Geometry: final body of the model. Coordinates: model frame, mm. Face numbers are marked on the shaded views. A direction names the side the tool comes from. Give positions to 0.01 mm unless a question says otherwise; leave off trailing zeros. Order: outer loops, then holes, each group sorted by start corner. A loop starts at its lowest first (then second) coordinate and runs counter-clockwise, first axis right, second up. Notation, with made-up numbers: (75, 79) -> (126, 79) arc R14 ccw to (126, 101) -> close; hole circle Ø1 at (-30.75, 48.25). An arc over 180 degrees is marked (long way). Write item = value, one per line.
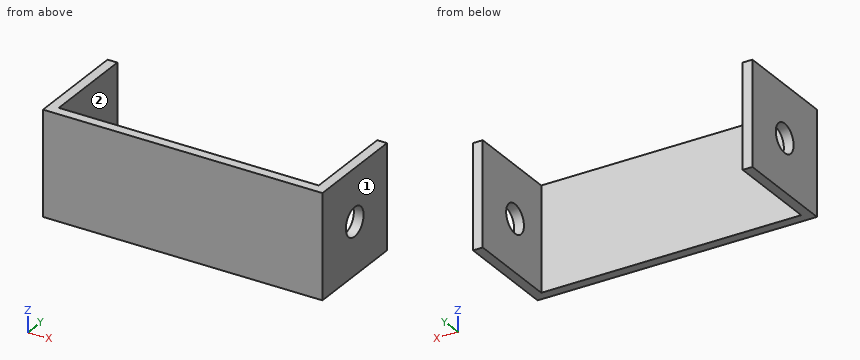
```python
from build123d import *

# Parameters (mm, degrees)
SKETCH1_W           = 127
SKETCH1_H           = 50.8
BOSS_EXTRUDE2_DEPTH = 4.7625
SKETCH3_W           = 4.7625
SKETCH3_H           = 50.8
BOSS_EXTRUDE3_DEPTH = 50.8
SKETCH4_R           = 6.985
CUT_EXTRUDE1_DEPTH  = 137.525


with BuildPart() as part:
    # Sketch1 → Boss-Extrude2 (new body)
    with BuildSketch(Plane(origin=(0, 0, 0), x_dir=(1, 0, 0), z_dir=(0, 1, 0))):
        with Locations((-6.634328358, 6.065671642)):
            Rectangle(SKETCH1_W, SKETCH1_H)
    extrude(amount=BOSS_EXTRUDE2_DEPTH)

    # Sketch3 → Boss-Extrude3 (add)
    with BuildSketch(Plane(origin=(0, 0, 0), x_dir=(1, 0, 0), z_dir=(0, 1, 0))):
        with Locations((59.246921642, 6.065671642)):
            Rectangle(SKETCH3_W, SKETCH3_H)
        with Locations((-72.515578358, 6.065671642)):
            Rectangle(SKETCH3_W, SKETCH3_H)
    extrude(amount=BOSS_EXTRUDE3_DEPTH)

    # Sketch4 → Cut-Extrude1 (cut, through all)
    with BuildSketch(Plane.ZY.offset(74.896828358)):
        with Locations((-6.065671642, 25.4)):
            Circle(SKETCH4_R)
    extrude(amount=-CUT_EXTRUDE1_DEPTH, mode=Mode.SUBTRACT)


solid = part.part
```
1) Reachability of the marked faces 1 and 2 from +Z, -Z, +X, -X, +Y, -Y: full face, straight path, thin tool, end or side. Return the list, or none.
Check sheet entries:
face_1 = +Z, -Z, +X, +Y, -Y
face_2 = +Z, -Z, +Y
2) Section query C-C (z = -4.5). Output: boundary loops of the cut face in (x, y).
Check sheet entries:
outline = (-74.9, 0) -> (61.63, 0) -> (61.63, 18.59) -> (56.87, 18.59) -> (56.87, 4.76) -> (-70.13, 4.76) -> (-70.13, 18.59) -> (-74.9, 18.59) -> close; (-74.9, 32.21) -> (-70.13, 32.21) -> (-70.13, 50.8) -> (-74.9, 50.8) -> close; (56.87, 32.21) -> (61.63, 32.21) -> (61.63, 50.8) -> (56.87, 50.8) -> close
3) Section query A-A (y = 7). Output: boundary loops of the cut face in (x, z), plus the area to 3 significant figures.
Check sheet entries:
outline = (-74.9, -31.47) -> (-70.13, -31.47) -> (-70.13, 19.33) -> (-74.9, 19.33) -> close; (56.87, -31.47) -> (61.63, -31.47) -> (61.63, 19.33) -> (56.87, 19.33) -> close
area = 484 mm²
4) Line query: line 1 (X direction, y = 37, z = 12); line 2 (Y direction, x = 26.5, z = -16). Output: solid intervals per line, ascending. Write a range as from..to.
Check sheet entries:
line_1 = -74.9..-70.13, 56.87..61.63
line_2 = 0..4.76
5) Section query D-D (z = 13). Output: boundary loops of the cut face in (x, y), plus the area to 3 significant figures.
Check sheet entries:
outline = (-74.9, 0) -> (61.63, 0) -> (61.63, 50.8) -> (56.87, 50.8) -> (56.87, 4.76) -> (-70.13, 4.76) -> (-70.13, 50.8) -> (-74.9, 50.8) -> close
area = 1,090 mm²
6) First-contact query: P1, Ø8, axis at x = 48, z = 7.5, coming from the +Y side. Flat tip, straight axial feed; report the tip coordinate or a pass-through.
Check sheet entries:
P1 = 4.76
7) Section query B-B (y = 25.4). Output: boundary loops of the cut face in (x, z).
Check sheet entries:
outline = (-74.9, -31.47) -> (-70.13, -31.47) -> (-70.13, -13.05) -> (-74.9, -13.05) -> close; (-74.9, 0.92) -> (-70.13, 0.92) -> (-70.13, 19.33) -> (-74.9, 19.33) -> close; (56.87, -31.47) -> (61.63, -31.47) -> (61.63, -13.05) -> (56.87, -13.05) -> close; (56.87, 0.92) -> (61.63, 0.92) -> (61.63, 19.33) -> (56.87, 19.33) -> close
